from build123d import *

# Parameters (mm, degrees)
SKETCH_1_R               = 15
EXTRUDE_1_DEPTH          = 45
SKETCH_2_R               = 11
CUT_EXTRUDE_1_DEPTH      = 40
SKETCH_3_R               = 7.5
CUT_EXTRUDE_2_DEPTH      = 5
SKETCH_4_W               = 3
SKETCH_4_H               = 15
EXTRUDE_2_DEPTH          = 30
SKETCH_5_R               = 1.75
CUT_EXTRUDE_3_DEPTH      = 30
SKETCH_6_R               = 1.75
CUT_EXTRUDE_4_DEPTH      = 30
SKETCH_7_R               = 1.75
CUT_EXTRUDE_5_DEPTH      = 30
SKETCH_8_R               = 1.75
CUT_EXTRUDE_6_DEPTH      = 10
PATTERN_CIRCULAR_1_COUNT = 3


with BuildPart() as part:
    # 草圖1 → 填料-伸長1 (new body)
    with BuildSketch(Plane.XY):
        Circle(SKETCH_1_R)
    extrude(amount=EXTRUDE_1_DEPTH)

    # 草圖2 → 除料-伸長1 (cut)
    with BuildSketch(Plane.XY.offset(45)):
        Circle(SKETCH_2_R)
    extrude(amount=-CUT_EXTRUDE_1_DEPTH, mode=Mode.SUBTRACT)

    # 草圖3 → 除料-伸長2 (cut)
    with BuildSketch(Plane.XY.offset(5)):
        Circle(SKETCH_3_R)
    extrude(amount=-CUT_EXTRUDE_2_DEPTH, mode=Mode.SUBTRACT)

    # 草圖4 → 填料-伸長2 (add)
    with BuildSketch(Plane.XY):
        Polygon((26.361016738, -13.487489302), (13.370635681, -5.987489302), (11.870635681, -8.585565513), (24.861016738, -16.085565513), align=None)
        with Locations((0, 22.073054816)):
            Rectangle(SKETCH_4_W, SKETCH_4_H)
        Polygon((-24.861016738, -16.085565513), (-11.870635681, -8.585565513), (-13.370635681, -5.987489302), (-26.361016738, -13.487489302), align=None)
    extrude(amount=EXTRUDE_2_DEPTH)

    # 草圖5 → 除料-伸長3 (cut)
    with BuildSketch(Plane(origin=(-0.75, -1.299038106, 0), x_dir=(0.866025404, -0.5, 0), z_dir=(-0.5, -0.866025404, 0))):
        with Locations((23.573054816, 15)):
            Circle(SKETCH_5_R)
    extrude(amount=-CUT_EXTRUDE_3_DEPTH, mode=Mode.SUBTRACT)

    # 草圖6 → 除料-伸長4 (cut)
    with BuildSketch(Plane(origin=(1.5, 0, 0), x_dir=(0, 0, -1), z_dir=(1, 0, 0))):
        with Locations((-15, 23.573054816)):
            Circle(SKETCH_6_R)
    extrude(amount=-CUT_EXTRUDE_4_DEPTH, mode=Mode.SUBTRACT)

    # 草圖7 → 除料-伸長5 (cut)
    with BuildSketch(Plane(origin=(-0.75, 1.299038106, 0), x_dir=(0.866025404, 0.5, 0), z_dir=(-0.5, 0.866025404, 0))):
        with Locations((-23.573054816, -15)):
            Circle(SKETCH_7_R)
    extrude(amount=-CUT_EXTRUDE_5_DEPTH, mode=Mode.SUBTRACT)

    # 草圖8 → 除料-伸長6 (cut)
    with BuildSketch(Plane(origin=(0, -15, 0), x_dir=(0, 0, -1), z_dir=(0, -1, 0))):
        with Locations((-25, 0)):
            Circle(SKETCH_8_R)
    cut_extrude_6 = extrude(amount=-CUT_EXTRUDE_6_DEPTH, mode=Mode.SUBTRACT)

    # 環狀複製排列1: 除料-伸長6 ×3 about axis
    pattern_circular_1_axis = Axis((0, 0, 0), (0, 0, 1))
    for i in range(1, PATTERN_CIRCULAR_1_COUNT):
        add(cut_extrude_6.rotate(pattern_circular_1_axis, i * 360 / PATTERN_CIRCULAR_1_COUNT), mode=Mode.SUBTRACT)


solid = part.part
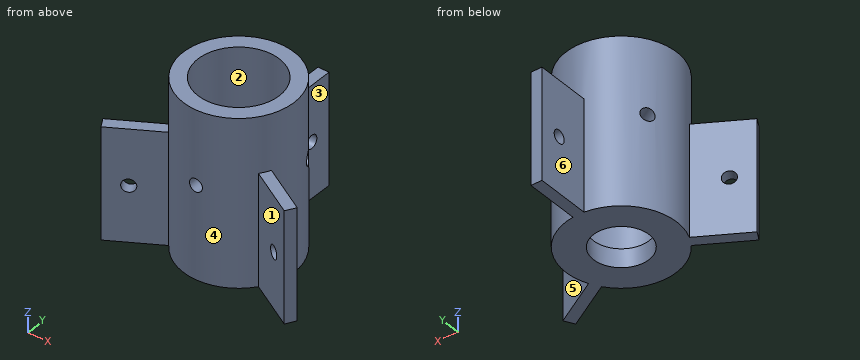
Model file for the job. Use its own axes, mm. Face numbers are marked on the shaded views. A direction names the side the tool comes from. Give positions to 0.01 mm unless a question says otherwise; leave off trailing zeros. Write each loop counter-clockwise with the first axis right and the second up, starting at its lowest first coordinate (ties: lowest second). Pieces come first, ordered by that corner, then holes. Notation, with made-up numbers: (58, -25.5) -> (82, -25.5) arc R21 ccw to (82, -13.5) -> close; hole circle Ø7 at (-35.5, 49). An arc over 180 degrees is marked (long way). Write item = value, one per line.
(1) Slice it at B-B, the plane x = 0. Give the cut face in (y, z).
Determined:
outline = (-15, 0) -> (-7.5, 0) -> (-7.5, 5) -> (-11, 5) -> (-11, 23.25) -> (-15, 23.25) -> close; (-15, 26.75) -> (-11, 26.75) -> (-11, 45) -> (-15, 45) -> close; (7.5, 0) -> (29.57, 0) -> (29.57, 30) -> (15, 30) -> (15, 45) -> (11, 45) -> (11, 5) -> (7.5, 5) -> close; hole circle Ø3.5 at (23.57, 15)
(2) Mould opens along X. For the marked faces 4, 5 and 6 say: released by +X, released by -X, zero draft, split by the parting line, or undercut.
Determined:
face_4 = undercut
face_5 = released by +X
face_6 = released by -X
(3) Slice it at D-D, the plane z = 15. Give the cut face in (x, y).
Determined:
outline = (-26.36, -13.49) -> (-24.86, -16.09) -> (-21.18, -13.96) -> (-22.68, -11.36) -> close; (-19.65, -9.61) -> (-18.15, -12.21) -> (-12.18, -8.76) arc R15 ccw to (12.18, -8.76) -> (18.15, -12.21) -> (19.65, -9.61) -> (13.68, -6.16) arc R15 ccw to (1.5, 14.92) -> (1.5, 21.82) -> (-1.5, 21.82) -> (-1.5, 14.92) arc R15 ccw to (-13.68, -6.16) -> close; (-1.5, 25.32) -> (1.5, 25.32) -> (1.5, 29.57) -> (-1.5, 29.57) -> close; (21.18, -13.96) -> (24.86, -16.09) -> (26.36, -13.49) -> (22.68, -11.36) -> close; hole circle Ø22 at (0, 0)
(4) Slice it at A-A, the plane z = 9. Give the cut face in (x, y).
Determined:
outline = (-26.36, -13.49) -> (-24.86, -16.09) -> (-12.18, -8.76) arc R15 ccw to (12.18, -8.76) -> (24.86, -16.09) -> (26.36, -13.49) -> (13.68, -6.16) arc R15 ccw to (1.5, 14.92) -> (1.5, 29.57) -> (-1.5, 29.57) -> (-1.5, 14.92) arc R15 ccw to (-13.68, -6.16) -> close; hole circle Ø22 at (0, 0)
(5) Probe line 1 along Y through (x, z) = (-0.05, 15); line 2 along Y through (x, z) = (0, 35); line 3 along X through (y, z) = (-12, 11). List the from-to ranges inside material, lowest first.
Determined:
line_1 = -15 to -11, 11 to 21.82, 25.32 to 29.57
line_2 = -15 to -11, 11 to 15
line_3 = -23.78 to -17.78, -9 to 9, 17.78 to 23.78
(6) Flat gauge pins, fed straight in: P1, Ø1.5, axis at x = 0.5, y = 22.5, coming from the +Z side; P2, Ø2, axis at y = -3, z = 22.5, coming from the +X side; P3, Ø4.5, axis at y = 23.57, z = 15, coming from the -X side. Where does each tip first touch, or does it go through?
Determined:
P1 = 30
P2 = 14.87
P3 = -1.5
(7) Slice it at C-C, the plane y = 0. Give the cut face in (x, z).
Determined:
outline = (-15, 0) -> (-7.5, 0) -> (-7.5, 5) -> (-11, 5) -> (-11, 45) -> (-15, 45) -> close; (7.5, 0) -> (15, 0) -> (15, 45) -> (11, 45) -> (11, 5) -> (7.5, 5) -> close
(8) Tool access for the marked faces 1, 2 and 3: list every direction of +Z, -Z, +X, -X, +Y, -Y with a clear straight run to the whole face (end or side of a thin tool).
Determined:
face_1 = +Z, -Z, -Y
face_2 = +Z
face_3 = +Z, -Z, +X, +Y
